Autodesk Fusion 360 part; units mm, degrees
sketch "Sketch1" plane through (0, 0, 0) normal (0, 0, 1) x (1, 0, 0)
  circle A0 centre (0, 0) radius 42.5
  dimension "d1" = 85
extrude "Extrude1" add sketch "Sketch1" along normal blind 7.5 makes body 1
sketch "Sketch2" plane through (0, 0, 7.5) normal (0, 0, 1) x (-1, 0, 0)
  circle A0 centre (0, 0) radius 42.5
  circle A1 centre (0, 0) radius 40
extrude "Extrude2" add sketch "Sketch2" along normal blind 5 draft -75 contours A1 bodies 1
sketch "Sketch3" plane through (0, 0, 12.5) normal (0, 0, 1) x (-1, 0, 0)
  circle A0 centre (0, 0) radius 21.3397
extrude "Extrude3" add sketch "Sketch3" along normal blind 12 draft -25 bodies 1
extrude "Extrude4" add 1 faces at (-1.9173, -4.8852, 24.5) along direction (0, 0, 1) blind 5 draft 5 on bodies 1 bodies 1
sketch "Sketch4" plane through (0, 0, 0) normal (0, 1, 0) x (1, 0, 0)
sketch "Sketch5" plane through (0, 0, 29.5) normal (0, 0, 1) x (-1, 0, 0)
  circle A0 centre (0, 0) radius 16.1815
  circle A1 centre (0, 0) radius 17.35
  dimension "d10" = 34.7
extrude "Extrude5" add sketch "Sketch5" along normal blind 2 separate body makes body 2
extrude "Extrude6" add 1 faces at (1.2002, -5.2586, 29.5) along direction (0, 0, 1) blind 2 on bodies 1 bodies 1 2
sketch "Sketch6" plane through (0, 0, 0) normal (0, 0, -1) x (1, 0, 0)
  circle A0 centre (0, 0) radius 42.5
  circle A1 centre (0, 0) radius 38.3224
extrude "Extrude7" cut sketch "Sketch6" against normal blind 5 contours A1 bodies 1
For this review, take the finished solid that the model builds, in its own axes (mm). A direction names the side the tool comes from. Coordinates: 2 decimals unless noted, no trailing zeros. Write each loop counter-clockwise with the first axis right and the second up, starting at its lowest first coordinate (ties: lowest second). Pieces come first, ordered by that corner, then holes.
(1) Add section C-C on z = 11. Give the boundary of the cut face in (x, y).
(2) Wall thickness on probe 1 along Y at (x, z) = (0, 2.1); probe 2 along Z at (x, y) = (36, -21); probe 3 along Y at (x, z) = (-28.5, 2.5): over which ranges is each line inside the solid? List them lowest first.
(3) For pin 1 Ø17.5 at (x, y) = (0, 3) entering from -Z; pin 2 Ø8 at (y, z) = (-0.5, 21.5) entering from -X; pin 3 Ø6 at (x, z) = (28.5, 6.5) entering from +Y; pin 4 Ø10 at (x, y) = (-28.5, 25) entering from -Z, all flat-tipped, find the tip position at first contact; note any pin that passes through.
(4) Add section D-D on z = 17. Give the boundary of the cut face in (x, y).
(5) Add section A-A on x = 0. Give the boundary of the cut face in (y, z).
(6) The part is to be moulded in two halves that separate along Z. For faces 1 (the face through (-5, -16, 29.5)), 2 (the face through (4.879, -21.972, 12.187)), 3 (the face through (-4.989, -37.996, 2.465)), say which applies: +Z half, -Z half, draft (parallel to the pull), parting line (faces both ways), or undercut.
(7) Tool access review of faces 4 (the face through (2.259, 17.202, 30.486)), 5 (the face through (3.44, 15.49, 25.92)), 6 (the face through (-6.5, 38, 0)), 7 (the face through (-1, -1, 5)), 8 (the face through (-33.727, 25.861, 3.698)): name each direction out of +Z, -Z, +X, -X, +Y, -Y from which nothing blocks a thin tool from reaching the whole face with its end or side.
Answer sheet:
1. outline: circle Ø53.88 at (0, 0)
2. probe 1: y = -42.5 to -38.32, 38.32 to 42.5
2. probe 2: z = 0 to 7.5
2. probe 3: y = -31.53 to -25.62, 25.62 to 31.53
3. pin 1: stops at z = 5
3. pin 2: stops at x = -19
3. pin 3: stops at y = 34
3. pin 4: stops at z = 0
4. outline: circle Ø38.48 at (0, 0)
5. outline: (-42.5, 0) - (-38.32, 0) - (-38.32, 5) - (38.32, 5) - (38.32, 0) - (42.5, 0) - (42.5, 7.5) - (40, 7.5) - (21.34, 12.5) - (15.74, 24.5) - (16.18, 29.5) - (17.35, 29.5) - (17.35, 31.5) - (-17.35, 31.5) - (-17.35, 29.5) - (-16.18, 29.5) - (-15.74, 24.5) - (-21.34, 12.5) - (-40, 7.5) - (-42.5, 7.5) - close
6. face 1: undercut
6. face 2: +Z half
6. face 3: draft
7. face 4: +Z
7. face 5: none
7. face 6: -Z, +X, -X, +Y, -Y
7. face 7: -Z
7. face 8: +Z, -Z
